from build123d import *

# Parameters (mm, degrees)
EXTRUDE_1_DEPTH             = 6.5
HOLE_WIZARD_M61_D           = 5
HOLE_WIZARD_M61_CSINK_D     = 6.05
HOLE_WIZARD_M61_CSINK_ANGLE = 90
FILLET_1_R                  = 0.3


with BuildPart() as part:
    # Эскиз1 → Бобышка-Вытянуть1 (new body, symmetric)
    with BuildSketch(Plane.XY):
        with BuildLine():
            Line((-3, 0), (3, 0))
            Line((3, 0), (3, -0.8))
            Line((3, -0.8), (4, -0.8))
            Line((4, -0.8), (4, -1.4))
            Line((4, -1.4), (1.536396103, -3.863603897))
            ThreePointArc((1.536396103, -3.863603897), (0, -4.5), (-1.536396103, -3.863603897))
            Line((-1.536396103, -3.863603897), (-4, -1.4))
            Line((-4, -1.4), (-4, -0.8))
            Line((-4, -0.8), (-3, -0.8))
            Line((-3, -0.8), (-3, 0))
        make_face()
    extrude(amount=EXTRUDE_1_DEPTH, both=True)

    # Отверстие обработанное метчиком M61 (through all)
    with Locations(Plane(origin=(0, 0, 0), x_dir=(1, 0, 0), z_dir=(0, 1, 0))):
        with Locations((0, -2)):
            CounterSinkHole(HOLE_WIZARD_M61_D / 2, HOLE_WIZARD_M61_CSINK_D / 2, counter_sink_angle=HOLE_WIZARD_M61_CSINK_ANGLE)

    # Эскиз5 → Повернуть1 (revolve)
    with BuildSketch(Plane(origin=(0, 0, 0), x_dir=(0, 0, -1), z_dir=(1, 0, 0))):
        with BuildLine():
            Line((4, -2), (4, -5))
            ThreePointArc((4, -5), (2.5, -3.5), (4, -2))
        make_face()
    revolve(axis=Axis((0, -2, -4), (0, -1, 0)))

    # Скругление1
    fillet_1_edges = [part.edges().sort_by_distance(p)[0] for p in [
        (4, -0.8, 0),
        (4, -1.4, 0),
        (-4, -1.4, 0),
        (-4, -0.8, 0),
    ]]
    fillet(fillet_1_edges, radius=FILLET_1_R)


solid = part.part
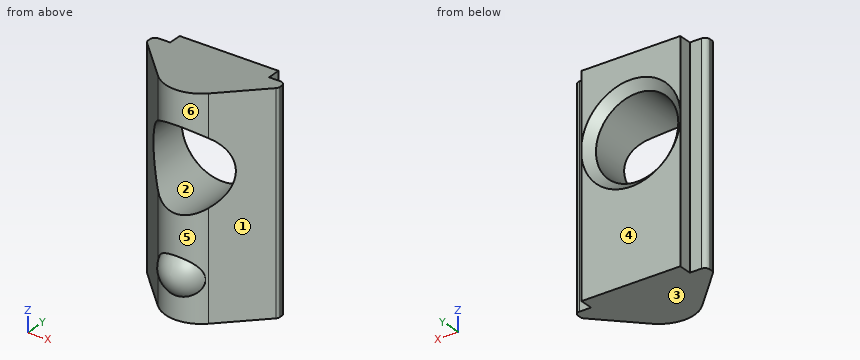
Can you work these out from the model? Positions are in its coordinate system, mm. Face numbers are marked on the shaded views. A direction names the side the tool comes from. Give positions to 0.01 mm unless a question says otherwise; leave off trailing zeros. Order: outer loops, then holes, each group sorted by start corner. A loop starts at its lowest first (then second) coordinate and runs counter-clockwise, first axis right, second up. Notation, with made-up numbers: M 3.5,77 L 58.5,77 A23 cw 58.5,116 Z; hole C 79,50 d1. An arc over 180 degrees is marked long. Use a Markdown table: item, result. Add a question column.
Item 1: Will these pins go through, and if not, where does the flat tip stop? pin 1 (4.5 mm diameter, centred on x = 0, z = 2, fed in from -Y); pin 2 (1.5 mm diameter, centred on y = -3.5, z = -2, fed in from -X).
Item 2: Suppose I cut it at D-D (z = 2). List the corners of the cut face in (x, y) for me (3 decimals).
Item 3: If I drill on L1, parallel to Z at x = 0, y = -3.9; L2, parallel to Z at x = 1.5, y = -2.55; L3, parallel to Y at x = 0, z = -2.5, over which ranges is the centre line in solid material (lowest first)? Write a range as [from, to].
Item 4: Suppose I cut it at B-B (y = -1.9). List the corners of the cut face in (x, z) for me, then the cut area to 3 significant figures.
Item 5: Suppose I cut it at C-C (z = 5.25). List the corners of the cut face in (x, y) for me, then the cut area to 3 significant figures.
Item 6: Suppose I cut it at A-A (x = 0). List the corners of the cut face in (y, z) for me (3 decimals), then the cut area to 3 significant figures.
Item 7: We'd pull the mould along Z, two halves only. Please class the marked faces 1, 2 and 3: +Z half, -Z half, draft (parallel to the pull), parting line (faces both ways), or undercut.
Item 8: For the marked faces 4, 5 and 6, which set-ups out of +Z, -Z, +X, -X, +Y, -Y let a thin tool reach every point of the face, with its end or its side?
Answer sheet:
| question | item | result |
|---|---|---|
| 1 | pin 1 | passes through |
| 1 | pin 2 | stops at x = -2.65 |
| 2 | outline | M -4,-1.276 A0.3 ccw -3.912,-1.488 L -2.5,-2.9 L -2.5,-0.525 L -3,-0.025 L -3,-0.8 L -3.7,-0.8 A0.3 ccw -4,-1.1 Z; M 2.5,-2.9 L 3.912,-1.488 A0.3 ccw 4,-1.276 L 4,-1.1 A0.3 ccw 3.7,-0.8 L 3,-0.8 L 3,-0.025 L 2.5,-0.525 Z |
| 3 | L1 | z = [-6.5, -0.5], [4.5, 6.5] |
| 3 | L2 | z = [-6.5, 0], [4, 6.5] |
| 3 | L3 | y = [-4.5, 0] |
| 4 | outline | M -3.5,-6.5 L 3.5,-6.5 L 3.5,6.5 L -3.5,6.5 Z; hole C 0,2 d5 |
| 4 | area | 71.4 mm² |
| 5 | outline | M -4,-1.28 A0.3 ccw -3.91,-1.49 L -1.54,-3.86 A2.17 ccw 1.54,-3.86 L 3.91,-1.49 A0.3 ccw 4,-1.28 L 4,-1.1 A0.3 ccw 3.7,-0.8 L 3,-0.8 L 3,0 L -3,0 L -3,-0.8 L -3.7,-0.8 A0.3 ccw -4,-1.1 Z |
| 5 | area | 24.5 mm² |
| 6 | outline | M -4.5,-6.5 L 0,-6.5 L 0,-1.025 L -0.525,-0.5 L -4.5,-0.5 L -4.5,-2.882 A1.5 ccw -4.5,-5.118 Z; M -4.5,4.5 L -0.525,4.5 L 0,5.025 L 0,6.5 L -4.5,6.5 Z |
| 6 | area | 36.5 mm² |
| 7 | face 1 | draft |
| 7 | face 2 | undercut |
| 7 | face 3 | -Z half |
| 8 | face 4 | +Z, -Z, +X, -X, +Y |
| 8 | face 5 | -Y |
| 8 | face 6 | +Z, -Y |
